Autodesk Inventor part; units mm, degrees
ref_plane "YZ Plane" through (0, 0, 0) normal (1, 0, 0) x (0, 1, 0)
ref_plane "XZ Plane" through (0, 0, 0) normal (0, 1, 0) x (-1, 0, 0)
ref_plane "XY Plane" through (0, 0, 0) normal (0, 0, 1) x (1, 0, 0)
sketch "Sketch1" plane through (0, 0, 0) normal (0, 0, 1) x (1, 0, 0)
  circle A0 centre (-76.4616, -331.0553) radius 285.0725
  line L0 (42.2033, -71.8546) -> (14.6776, -21.3711)
  line L1 (14.6776, -21.3711) -> (-35.8059, -48.8968)
  line L2 (-35.8059, -48.8968) -> (-37.0027, -46.7018)
  line L3 (-37.0027, -46.7018) -> (15.6758, -17.9794)
  line L4 (15.6758, -17.9794) -> (44.3982, -70.6579)
  line L5 (44.3982, -70.6579) -> (42.2033, -71.8546)
  dimension "d15" = 2.5
  dimension "d16" = 60
extrude "Extrusion1" add sketch "Sketch1" along normal mid plane 1100 contours L0 L1 L2 L3 L4 L5
sketch "Sketch3" plane through (0, 0, 0) normal (0, 0, 1) x (1, 0, 0)
  circle A0 centre (3.5411, -59.2122) radius 5
  circle A1 centre (3.5411, -59.2122) radius 10
  line L0 (-35.8059, -48.8968) -> (14.6776, -21.3711)
  line L1 (14.6776, -21.3711) -> (42.2033, -71.8546)
  line L2 (8.3282, -67.992) -> (32.817, -54.6397)
  line L3 (32.817, -54.6397) -> (18.1516, -27.7427)
  line L4 (18.1516, -27.7427) -> (8.3061, -24.8451)
  line L5 (8.3061, -24.8451) -> (-18.591, -39.5105)
  line L6 (-18.591, -39.5105) -> (-5.2387, -63.9993)
  point P0 (0, 0)
  dimension "d21" = 10
  dimension "d22" = 20
extrude "Extrusion4" add sketch "Sketch3" along normal mid plane 6 contours A1 | A1 L6 L0 L4 L1 L2
properties part number "Barra freno"
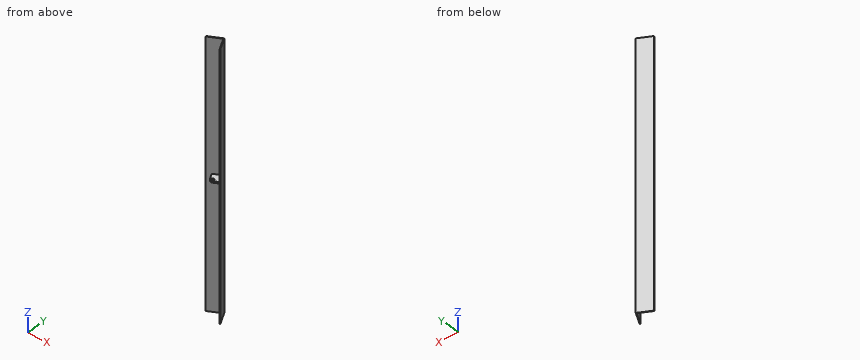
Could you check a few things on this model? Use its own coordinates, in mm. Coordinates: 2 decimals unless noted, no trailing zeros. Loops run counter-clockwise (first coordinate to the right, second up) from the corner with the lowest first, then second, coordinate; pieces in that order, holes last.
1. For P1, Ø13, axis at x = 3.54, y = -59.21, coming from the +Z side; P2, Ø2, axis at y = -31, z = -356, coming from the -X side; P3, Ø1.5, axis at x = 6, z = 196, coming from the +Y side, each with a flat end and sliding along its axis, tell me the tip position at first contact or that it passes through.
2. Imagine slicing it at A-A (z = -200.5). Please give me the cut outline in (x, y), and give its area (3 significant figures).
3. I need wall thicknesses on L1, parallel to Z at x = -5, y = -50.5; L2, parallel to X at y = -30, z = -171.5; L3, parallel to X at y = -28.5, z = -417.5. Which ranges of each line are inside material? Lowest first, please.
Computed values:
1. P1: stops at z = 3
1. P2: stops at x = -10.04
1. P3: stops at y = -22.85
2. outline: (-37, -46.7) - (-35.81, -48.9) - (14.68, -21.37) - (42.2, -71.85) - (44.4, -70.66) - (15.68, -17.98) - close
2. area: 294 mm2
3. L1: z = -3 to 3
3. L2: x = -6.37 to -1.15, 19.38 to 22.23
3. L3: x = -3.62 to 1.6, 18.56 to 21.41
